Here's how the part is built. I have some questions about the finished solid (model axes, mm). A direction names the side the tool comes from. Coordinates: 2 decimals unless noted, no trailing zeros. Loops run counter-clockwise (first coordinate to the right, second up) from the corner with the lowest first, then second, coordinate; pieces in that order, holes last. Notation, with made-up numbers: (60.5, 36.5) - (89.5, 36.5) arc R30 cw to (89.5, 65.5) - close; hole circle Ø8 at (47, 35). An arc over 180 degrees is marked (long way). Use a Markdown table: item, result.
```python
from build123d import *

# Parameters (mm, degrees)
SKETCH1_W           = 50
SKETCH1_H           = 2
BOSS_EXTRUDE1_DEPTH = 2
SKETCH6_W           = 35
SKETCH6_H           = 2
CUT_EXTRUDE1_DEPTH  = 2


with BuildPart() as part:
    # Sketch1 → Boss-Extrude1 (new body)
    with BuildSketch(Plane(origin=(0, 0, 0), x_dir=(1, 0, 0), z_dir=(0, 1, 0))):
        with BuildLine():
            Line((-120.405540847, 10.840369707), (-64.990311195, 15.45833074))
            Line((-64.990311195, 15.45833074), (-54.990311195, 5.45833074))
            Line((-54.990311195, 5.45833074), (-44.990311195, 5.45833074))
            Line((-44.990311195, 5.45833074), (-44.990311195, 15.45833074))
            Line((-44.990311195, 15.45833074), (90.009688805, 4.0256009))
            Line((90.009688805, 4.0256009), (108.952709235, 34.277770331))
            ThreePointArc((108.952709235, 34.277770331), (111.494770003, 36.686709078), (114.88557379, 37.562784709))
            Line((114.88557379, 37.562784709), (118.009688805, 37.562784709))
            ThreePointArc((118.009688805, 37.562784709), (122.959436273, 35.512532177), (125.009688805, 30.562784709))
            Line((125.009688805, 30.562784709), (125.009688805, 15.562784709))
            Line((125.009688805, 15.562784709), (125.009688805, -5.9743991))
            Line((125.009688805, -5.9743991), (110.009688805, -5.9743991))
            Line((110.009688805, -5.9743991), (-19.990311195, -14.651713609))
            Line((-19.990311195, -14.651713609), (-69.990311195, -14.651713609))
            Line((-69.990311195, -14.651713609), (-120.534992278, -9.112602605))
            ThreePointArc((-120.534992278, -9.112602605), (-123.713441962, -7.479767666), (-124.990311195, -4.142358897))
            Line((-124.990311195, -4.142358897), (-124.990311195, 5.857641103))
            ThreePointArc((-124.990311195, 5.857641103), (-123.669723394, 9.243187717), (-120.405540847, 10.840369707))
        make_face()
        with Locations((-44.990311195, -4.651713609)):
            Rectangle(SKETCH1_W, SKETCH1_H, mode=Mode.SUBTRACT)
    extrude(amount=BOSS_EXTRUDE1_DEPTH)

    # Sketch6 → Cut-Extrude1 (cut)
    with BuildSketch(Plane(origin=(0, 2, 0), x_dir=(1, 0, 0), z_dir=(0, 1, 0))):
        with Locations((90.009688805, -1.362235571)):
            Rectangle(SKETCH6_W, SKETCH6_H)
    extrude(amount=-CUT_EXTRUDE1_DEPTH, mode=Mode.SUBTRACT)


solid = part.part
```
Q1. I want a section at C-C, the plane x = -33. Write out the boundary of the cut face in (y, z), then the cut area to 3 significant figures.
Check values:
| item | result |
|---|---|
| outline | (0, -14.44) - (2, -14.44) - (2, 3.65) - (0, 3.65) - close; (0, 5.65) - (2, 5.65) - (2, 14.65) - (0, 14.65) - close |
| area | 54.2 mm^2 |
Q2. Will these pins go through, and if not, where does the flat tip stop? P1, Ø0.6, axis at y = 1, z = 5, coming from the -X side; P2, Ø0.6, axis at x = 97, y = 1.5, coming from the +Z side; P3, Ø1, axis at x = 88, y = 0.5, coming from the -Z side.
Check values:
| item | result |
|---|---|
| P1 | x = -124.96 |
| P2 | z = 6.86 |
| P3 | z = -4.24 |
Q3. Please list where these lines run through material, in increasing order: L1, parallel to X at y = 1.05, z = 2; L2, parallel to X at y = 1.1, z = 5.5; L3, parallel to Z at x = 85, y = 1.95. Write a range as from..to.
Check values:
| item | result |
|---|---|
| L1 | -124.99..72.51, 107.51..125.01 |
| L2 | -124.8..-69.99, -19.99..125.01 |
| L3 | -4.45..0.36, 2.36..7.64 |
Q4. Which directions (+Z, -Z, +X, -X, +Y, -Y) give clear straight access to the entire face, cutting with the end or side of a thin tool? Please do faces 5 (the face through (99.35, 0.99, -18.94)), 6 (the face through (-93.086, 0.986, -13.117)).
Check values:
| item | result |
|---|---|
| face 5 | -Z, +Y, -Y |
| face 6 | -Z, -X, +Y, -Y |
Q5. I want a section at A-A, the plane y = 1.7. Write out the boundary of the cut face in (x, z) (3 decimals), then the cut area to 3 significant figures.
Check values:
| item | result |
|---|---|
| outline | (-124.99, -5.858) arc R5 ccw to (-120.406, -10.84) - (-64.99, -15.458) - (-54.99, -5.458) - (-44.99, -5.458) - (-44.99, -15.458) - (90.01, -4.026) - (108.953, -34.278) arc R7 ccw to (114.886, -37.563) - (118.01, -37.563) arc R7 ccw to (125.01, -30.563) - (125.01, 5.974) - (110.01, 5.974) - (-19.99, 14.652) - (-69.99, 14.652) - (-120.535, 9.113) arc R5 ccw to (-124.99, 4.142) - close; hole (-69.99, 3.652) - (-19.99, 3.652) - (-19.99, 5.652) - (-69.99, 5.652) - close; hole (72.51, 0.362) - (107.51, 0.362) - (107.51, 2.362) - (72.51, 2.362) - close |
| area | 5,830 mm^2 |
Q6. If we mould it in two halves opening along X, with no side actions, what happens to faces 1 (the face through (2, 0, 0)), 2 (the face through (-60.06, 0.99, -10.53)), 3 (the face through (21.565, 0.986, -9.822)), 4 (the face through (-94.91, 0.99, 11.92))? For each: pulls with the +X half, pulls with the -X half, needs draft (parallel to the pull), parting line crosses it, or undercut.
Check values:
| item | result |
|---|---|
| face 1 | needs draft |
| face 2 | undercut |
| face 3 | undercut |
| face 4 | pulls with the -X half |
Q7. I want a section at B-B, the plane x = 104. Write out the boundary of the cut face in (y, z).
Check values:
| item | result |
|---|---|
| outline | (0, -26.37) - (2, -26.37) - (2, 0.36) - (0, 0.36) - close; (0, 2.36) - (2, 2.36) - (2, 6.38) - (0, 6.38) - close |
Q8. I want a section at D-D, the plane x = -110. Write out the boundary of the cut face in (y, z), then the cut area to 3 significant figures.
Check values:
| item | result |
|---|---|
| outline | (0, -11.71) - (2, -11.71) - (2, 10.27) - (0, 10.27) - close |
| area | 43.9 mm^2 |
